from build123d import *

# Parameters (mm, degrees)
F0_W     = 20
F0_H     = 20
F0_R     = 2
F1_DEPTH = 20
F2_R     = 2
F3_DEPTH = 20.001
F4_R     = 2
F5_DEPTH = 20.001


with BuildPart() as f1:
    # F0 (on Top) → F1 (new body)
    with BuildSketch(Plane.XY):
        with Locations((10, -10)):
            Rectangle(F0_W, F0_H)
        with Locations((10, -10)):
            Circle(F0_R, mode=Mode.SUBTRACT)
    extrude(amount=F1_DEPTH)

    # F2 (on face) → F3 (cut, through all)
    with BuildSketch(Plane.YZ.offset(20)):
        with Locations((-10, 10)):
            Circle(F2_R)
    extrude(amount=-F3_DEPTH, mode=Mode.SUBTRACT)

    # F4 (on face) → F5 (cut, through all)
    with BuildSketch(Plane.XZ.offset(20)):
        with Locations((10, 10)):
            Circle(F4_R)
    extrude(amount=-F5_DEPTH, mode=Mode.SUBTRACT)


solid = f1.part
Verification items for the finished model (mm, model axes). Round coordinates to 2 decimals unless told otherwise and drop trailing zeros. Order: outer loops, then holes, each group sorted by start corner. A loop starts at its lowest first (then second) coordinate and runs counter-clockwise, first axis right, second up.
1. Section check A-A on x = 10. Record the cut outline in (y, z), then the cut area to 3 significant figures.
Final values:
outline: (-20, 0) - (-12, 0) - (-12, 8) - (-20, 8) - close; (-20, 12) - (-12, 12) - (-12, 20) - (-20, 20) - close; (-8, 0) - (0, 0) - (0, 8) - (-8, 8) - close; (-8, 12) - (0, 12) - (0, 20) - (-8, 20) - close
area: 256 mm2
2. Section check D-D on x = 3.25. Record the cut outline in (y, z), then the cut area to 3 significant figures.
Final values:
outline: (-20, 0) - (0, 0) - (0, 20) - (-20, 20) - close; hole circle Ø4 at (-10, 10)
area: 387 mm2
3. Section check C-C on y = -18. Record the cut outline in (x, z), then the cut area to 3 significant figures.
Final values:
outline: (0, 0) - (20, 0) - (20, 20) - (0, 20) - close; hole circle Ø4 at (10, 10)
area: 387 mm2
4. Thickness scan on L1, parallel to Y at x = 17.75, z = 10; L2, parallel to Z at x = 10, y = -2. Record the ranges inside material, lowest first.
Final values:
L1: y = -20 to -12, -8 to 0
L2: z = 0 to 8, 12 to 20
5. Section check B-B on z = 10. Record the cut outline in (x, y).
Final values:
outline: (0, -20) - (8, -20) - (8, -12) - (0, -12) - close; (0, -8) - (8, -8) - (8, 0) - (0, 0) - close; (12, -20) - (20, -20) - (20, -12) - (12, -12) - close; (12, -8) - (20, -8) - (20, 0) - (12, 0) - close
6. Release check for a two-part mould opening along X. For faces 1 (the flat face through (0, -12.4, 9.9)), 2 (the cylindrical face through (8, -4, 10)), 3 (the flat face through (9.9, -7.6, 0)) record: +X half, -X half, draft (parallel to the pull), parting line (faces both ways), or undercut.
Final values:
face 1: -X half
face 2: undercut
face 3: draft
